Verification items for the finished model (mm, model axes). Face numbers are marked on the shaded views. A direction names the side the tool comes from. Round coordinates to 2 decimals unless told otherwise and drop trailing zeros. Write each loop counter-clockwise with the first axis right and the second up, starting at its lowest first coordinate (ties: lowest second). Pieces come first, ordered by that corner, then holes. Notation, with made-up numbers: M -9.75,44.5 L 36.25,44.5 A22 ccw 36.25,56.5 Z; hole C 19,54 d6. An arc over 180 degrees is marked long. Answer in a Markdown table with one row per item. Add a question column.
1. Sectioned sample at B-B on x = -4.5. Record the cut outline in (y, z), plus the area to 3 significant figures.
2. Material ranges on probe 1 along Y at (x, z) = (0, 4); probe 2 along X at (y, z) = (-9.25, 8.5); probe 3 along X at (y, z) = (1.75, -0.5), recorded low to high.
3. Set-up check for the marked faces 1, 2, 3, 4 and 5: record each of +Z, -Z, +X, -X, +Y, -Y from which the full face is reachable in a straight line by a thin tool's end or side.
4. Sectioned sample at D-D on y = 10. Record the cut outline in (x, z), plus the area to 3 significant figures.
5. Go/stop test with flat-tipped pins: pin 1 Ø3 at (x, z) = (6.5, 9) entering from -Y; pin 2 Ø2 at (x, z) = (4, 7.5) entering from +Y; pin 3 Ø4.5 at (x, y) = (12.5, 2) entering from +Z. Record where each tip stops, or that it passes through.
6. Sectioned sample at C-C on z = 8. Record the cut outline in (x, y).
7. Sectioned sample at A-A on y = -0.5. Record the cut outline in (x, z), plus the area to 3 significant figures.
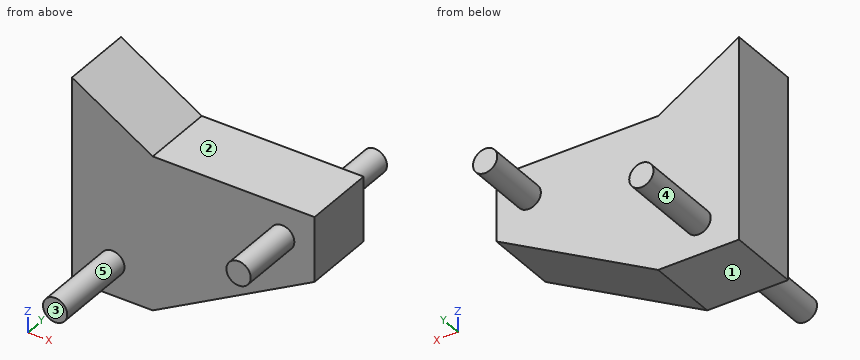
```python
from build123d import *

# Parameters (mm, degrees)
F0_R     = 1.5
F1_DEPTH = 4.5
F2_DEPTH = 15
F3_DEPTH = 12.5


with BuildPart() as f1:
    # F0 (on Front) → F1 (new body, symmetric)
    with BuildSketch(Plane.XZ):
        Polygon((-0.399913, 11.307418), (-10.399913, 17.307418), (-10.399913, -7.692582), (-0.399913, -7.692582), (19.600087, 3.307418), (19.600087, 11.307418), align=None)
        with Locations((-5.399913, -3.692582)):
            Circle(F0_R, mode=Mode.SUBTRACT)
        with Locations((15.600087, 7.307418)):
            Circle(F0_R, mode=Mode.SUBTRACT)
    extrude(amount=F1_DEPTH, both=True)

    # F0 (on Front) → F2 (join, symmetric)
    with BuildSketch(Plane.XZ):
        with Locations((-5.399913, -3.692582)):
            Circle(F0_R)
    extrude(amount=F2_DEPTH, both=True)

    # F0 (on Front) → F3 (join, symmetric)
    with BuildSketch(Plane.XZ):
        with Locations((15.600087, 7.307418)):
            Circle(F0_R)
    extrude(amount=F3_DEPTH, both=True)


solid = f1.part
```
Geometry check:
| question | item | result |
|---|---|---|
| 1 | outline | M -15,-4.89 L -4.5,-4.89 L -4.5,-7.69 L 4.5,-7.69 L 4.5,-4.89 L 15,-4.89 L 15,-2.49 L 4.5,-2.49 L 4.5,13.77 L -4.5,13.77 L -4.5,-2.49 L -15,-2.49 Z |
| 1 | area | 244 mm2 |
| 2 | probe 1 | y = -4.5 to 4.5 |
| 2 | probe 2 | x = 14.69 to 16.51 |
| 2 | probe 3 | x = -10.4 to 12.68 |
| 3 | face 1 | -Z, +X, -X, +Y, -Y |
| 3 | face 2 | +Z, +X, +Y, -Y |
| 3 | face 3 | +Z, -Z, +X, -X, -Y |
| 3 | face 4 | +Y |
| 3 | face 5 | -Y |
| 4 | outline | C -5.4,-3.69 d3; C 15.6,7.31 d3 |
| 4 | area | 14.1 mm2 |
| 5 | pin 1 | stops at y = -4.5 |
| 5 | pin 2 | stops at y = 4.5 |
| 5 | pin 3 | stops at z = 11.31 |
| 6 | outline | M -10.4,-4.5 L 14.27,-4.5 L 14.27,-12.5 L 16.93,-12.5 L 16.93,-4.5 L 19.6,-4.5 L 19.6,4.5 L 16.93,4.5 L 16.93,12.5 L 14.27,12.5 L 14.27,4.5 L -10.4,4.5 Z |
| 7 | outline | M -10.4,-7.69 L -0.4,-7.69 L 19.6,3.31 L 19.6,11.31 L -0.4,11.31 L -10.4,17.31 Z |
| 7 | area | 490 mm2 |
